from build123d import *

# Parameters (mm, degrees)
F0_R      = 17.145
F5_DEPTH  = 25.4
F1_R      = 8.255
F6_DEPTH  = 25.4
F2_R      = 2.413
F7_DEPTH  = 25.4
F9_SIZE   = 3.048
F10_SIZE  = 2.286
F8_R      = 5.08
F11_DEPTH = 25.4
F4_R      = 12.065
F12_DEPTH = 6.35
F13_SIZE  = 1.27


with BuildPart() as f5:
    # F0 (on Front) → F5 (new body)
    with BuildSketch(Plane.XZ):
        Circle(F0_R)
    extrude(amount=F5_DEPTH)

    # F1 (on Front) → F6 (join)
    with BuildSketch(Plane.XZ):
        Circle(F1_R)
    extrude(amount=-F6_DEPTH)

    # F2 (on Front) → F7 (cut)
    with BuildSketch(Plane.XZ):
        Circle(F2_R)
    extrude(amount=-F7_DEPTH, mode=Mode.SUBTRACT)

    # F9
    f9_edges = [f5.edges().sort_by_distance(p)[0] for p in [
        (-17.145, -25.4, 0),
    ]]
    chamfer(f9_edges, length=F9_SIZE)

    # F10
    f10_edges = [f5.edges().sort_by_distance(p)[0] for p in [
        (-17.145, 0, 0),
        (-8.255, 0, 0),
    ]]
    chamfer(f10_edges, length=F10_SIZE)

    # F8 (on Front) → F11 (cut)
    with BuildSketch(Plane.XZ):
        with Locations((0, 19.5638593286)):
            Circle(F8_R)
        with Locations((-16.9427991747, 9.7819296643)):
            Circle(F8_R)
        with Locations((-16.9427991747, -9.7819296643)):
            Circle(F8_R)
        with Locations((0, -19.5638593286)):
            Circle(F8_R)
        with Locations((16.9427991747, -9.7819296643)):
            Circle(F8_R)
        with Locations((16.9427991747, 9.7819296643)):
            Circle(F8_R)
    extrude(amount=F11_DEPTH, mode=Mode.SUBTRACT)

    # F4 (on offset) → F12 (cut)
    with BuildSketch(Plane.XZ.offset(25.4)):
        Circle(F4_R)
    extrude(amount=-F12_DEPTH, mode=Mode.SUBTRACT)

    # F13
    f13_edges = [f5.edges().sort_by_distance(p)[0] for p in [
        (-8.255, 25.4, 0),
    ]]
    chamfer(f13_edges, length=F13_SIZE)


solid = f5.part
The model under review builds one solid part; all positions refer to its coordinate system, in mm. A direction names the side the tool comes from. Give positions to 0.01 mm unless a question says otherwise; leave off trailing zeros. Loops run counter-clockwise (first coordinate to the right, second up) from the corner with the lowest first, then second, coordinate; pieces in that order, holes last. Notation, with made-up numbers: (53.25, 60) -> (66.25, 60) arc R10 cw to (66.25, 69) -> close; hole circle Ø7 at (18, -11.5). An arc over 180 degrees is marked (long way). Answer as a JSON object with one key per item and string values. Group by question number.
Q1. Take a section at B-B (x = 0). Write out the cut boundary in (y, z) (3 decimals).
Q2. Insertion check: pin 1 (12 mm diameter, centred on y = -2.5, z = -9, fed in from +X); pin 2 (5 mm diameter, centred on y = -13, z = -6.5, fed in from +X); pin 3 (2 mm diameter, centred on y = 7.5, z = 5.5, fed in from -X); pin 4 (4 mm diameter, centred on x = -0.5, z = 0, fed in from +Y). Each pin has a flat end and moves straight along its axis. Give the tip position at first contact, or say it passes through.
Q3. Take a section at A-A (z = 0). Write out the cut boundary in (x, y) (3 decimals).
Q4. Take a section at C-C (y = 7). Write out the cut boundary in (x, z) (3 decimals), plus the area to 3 significant figures.
Q5. Wall thickness on line 1 along Z through (x, y) = (0, -23.5) (3 decimals); line 2 along Z through (x, y) = (0, 10.5) (3 decimals); line 3 along Y through (x, z) = (-3, -12.5): over which ranges is each line inside the solid? List them lowest first.
Q6. Draft analysis for pull direction X (two halves, no side actions). For faces 3 (the flat face through (0, -19.05, 0)), 4 (the conical face through (-15.73, -0.87, 0.09)), 5 (the cylindrical face through (8.63, -12.179, 14.814)), state which applies: pulls with the +X half, pulls with the -X half, needs draft (parallel to the pull), parting line crosses it, or undercut.
Q7. Tool access review of faces 1 (the cylindrical face through (7.874, 13.055, 2.48)), 2 (the conical face through (13.59, -25.25, 4.28)): name each direction out of +Z, -Z, +X, -X, +Y, -Y from which nothing blocks a thin tool from reaching the whole face with its end or side.
Answer below:
{
 "1": {"outline": "(-25.4, -14.097) -> (-25.013, -14.484) -> (0, -14.484) -> (0, -10.541) -> (2.286, -8.255) -> (24.13, -8.255) -> (25.4, -6.985) -> (25.4, -2.413) -> (0, -2.413) -> (0, 2.413) -> (25.4, 2.413) -> (25.4, 6.985) -> (24.13, 8.255) -> (2.286, 8.255) -> (0, 10.541) -> (0, 14.484) -> (-25.013, 14.484) -> (-25.4, 14.097) -> (-25.4, 12.065) -> (-19.05, 12.065) -> (-19.05, -12.065) -> (-25.4, -12.065) -> close"},
 "2": {"pin 1": "stops at x = 16.88", "pin 2": "stops at x = 16.67", "pin 3": "stops at x = -6.92", "pin 4": "stops at y = 25.4"},
 "3": {"outline": "(-17.145, -22.352) -> (-14.097, -25.4) -> (-12.065, -25.4) -> (-12.065, -19.05) -> (12.065, -19.05) -> (12.065, -25.4) -> (14.097, -25.4) -> (17.145, -22.352) -> (17.145, -2.286) -> (14.859, 0) -> (10.541, 0) -> (8.255, 2.286) -> (8.255, 24.13) -> (6.985, 25.4) -> (2.413, 25.4) -> (2.413, 0) -> (-2.413, 0) -> (-2.413, 25.4) -> (-6.985, 25.4) -> (-8.255, 24.13) -> (-8.255, 2.286) -> (-10.541, 0) -> (-14.859, 0) -> (-17.145, -2.286) -> close"},
 "4": {"outline": "circle Ø16.51 at (0, 0); hole circle Ø4.826 at (0, 0)", "area": "196 mm2"},
 "5": {"line 1": "z = -14.484 to -12.065, 12.065 to 14.484", "line 2": "z = -8.255 to -2.413, 2.413 to 8.255", "line 3": "y = -25.4 to 0"},
 "6": {"face 3": "undercut", "face 4": "pulls with the -X half", "face 5": "pulls with the +X half"},
 "7": {"face 1": "+Y", "face 2": "-Y"}
}
